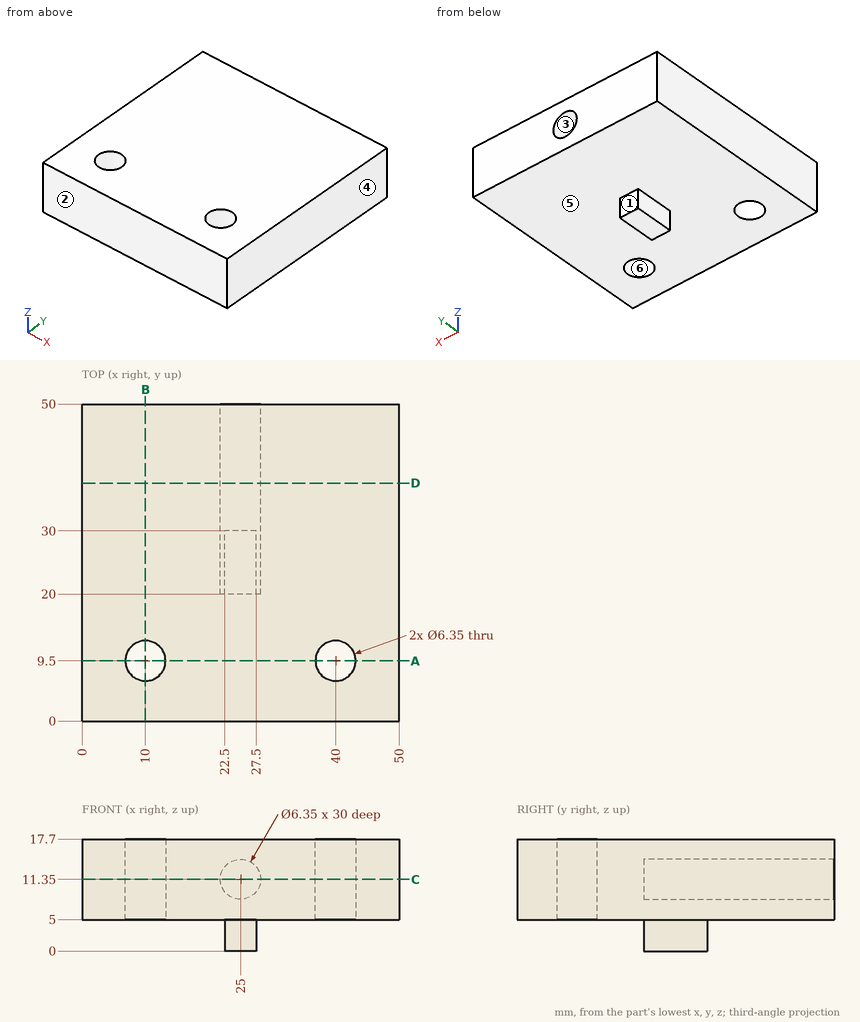
Geometry check sheet. Reference: drawing and pictorial views, mm from the part's lowest x, y, z. A direction names the side the tool comes from. Round coordinates to 2 decimals unless told otherwise and drop trailing zeros. Loops run counter-clockwise (first coordinate to the right, second up) from the corner with the lowest first, then second, coordinate; pieces in that order, holes last. Notation, with made-up numbers: (-6, 43) - (22, 43) arc R16 ccw to (22, 58) - close; hole circle Ø10 at (-36.75, -34.75). An arc over 180 degrees is marked (long way). One line per question, with ' | ' between items. Start each with the question number.
1. Cross-section at A-A on y = 9.5. Record the cut outline in (x, z) (3 decimals).
2. Scan lines: line 1 (Y direction, x = 10, z = 13) (3 decimals); line 2 (Z direction, x = 47, y = 34); line 3 (X direction, y = 31, z = 14.25). Record each from-to range of solid material in increasing order. Write a range as [from, to].
3. Depth check by flat-ended pin: pin 1 (1.9 mm diameter, centred on x = 24, z = 12, fed in from +Y); pin 2 (10 mm diameter, centred on x = 40, y = 9.5, fed in from -Z); pin 3 (1.5 mm diameter, centred on y = 26.5, z = 2.5, fed in from -X). Enter the tip coordinate at first touch or a pass-through.
4. Tool access check on the marked faces 1, 2 and 3. Record the directions out of +Z, -Z, +X, -X, +Y, -Y that give a thin tool (end or side, any length) a straight path to the whole face; none if there is none.
5. Cross-section at C-C on z = 11.35. Record the cut outline in (x, y) (3 decimals), then the cut area to 3 significant figures.
6. Draft check along X on the marked faces 4, 5 and 6. Enter one of: released by +X, released by -X, zero draft, split by the parting line, or undercut.
7. Cross-section at B-B on x = 10. Record the cut outline in (y, z) (3 decimals).
8. Cross-section at D-D on y = 37.5. Record the cut outline in (x, z) (3 decimals), then the cut area to 3 significant figures.
Taken from the geometry:
1) outline: (0, 5) - (6.825, 5) - (6.825, 17.7) - (0, 17.7) - close; (13.175, 5) - (36.825, 5) - (36.825, 17.7) - (13.175, 17.7) - close; (43.175, 5) - (50, 5) - (50, 17.7) - (43.175, 17.7) - close
2) line 1: [0, 6.325], [12.675, 50] | line 2: [5, 17.7] | line 3: [0, 23.71], [26.29, 50]
3) pin 1: y = 20 | pin 2: z = 5 | pin 3: x = 22.5
4) face 1: -Z, +X, -X, +Y | face 2: +Z, -Z, +X, -X, -Y | face 3: +Y
5) outline: (0, 0) - (50, 0) - (50, 50) - (28.175, 50) - (28.175, 20) - (21.825, 20) - (21.825, 50) - (0, 50) - close; hole circle Ø6.35 at (10, 9.5); hole circle Ø6.35 at (40, 9.5) | area: 2,250 mm²
6) face 4: released by +X | face 5: zero draft | face 6: undercut
7) outline: (0, 5) - (6.325, 5) - (6.325, 17.7) - (0, 17.7) - close; (12.675, 5) - (50, 5) - (50, 17.7) - (12.675, 17.7) - close
8) outline: (0, 5) - (50, 5) - (50, 17.7) - (0, 17.7) - close; hole circle Ø6.35 at (25, 11.35) | area: 603 mm²
